Drawing for the job (mm, zero at the part's lowest x, y, z). A direction names the side the tool comes from. Give positions to 0.01 mm unless a question says otherwise; leave off trailing zeros. Order: outer loops, then holes, each group sorted by start corner. A loop starts at its lowest first (then second) coordinate and runs counter-clockwise, first axis right, second up. Notation, with made-up numbers: (22.5, 82) -> (70.5, 82) arc R31 cw to (70.5, 107) -> close; hole circle Ø1 at (69.25, 83). An arc over 180 degrees is marked (long way). Use one line per item in the form item = value. Start each with the question number.
1) Drop flat-ended pins along their axis: P1, Ø3, axis at x = 35.5, z = 35.5, coming from the +Y side; P2, Ø1, axis at y = 1, z = 18.5, coming from the +X side. Give the stop position or say it passes through.
2) Mould opens along X. For the marked faces 1 and 2 say: pulls with the +X half, pulls with the -X half, needs draft (parallel to the pull), parting line crosses it, or undercut.
3) Probe line 1 (Z direction, x = 4.5, y = 1.4) (1 decimal); line 2 (X direction, y = 1.55, z = 3.5); line 3 (X direction, y = 0.65, z = 35.5) (1 decimal). List the from-to ranges inside material, lowest first.
4) Cut at C-C, the plane y = 4.7. Give the cut face in (x, z).
5) Cut at D-D, the plane y = 1.15. Give the cut face in (x, z).
6) Tool access for the marked faces 3, 4 and 5: list every direction of +Z, -Z, +X, -X, +Y, -Y with a clear straight run to the whole face (end or side of a thin tool).
7) Cut at A-A, the plane x = 20. Give the cut face in (y, z), and give its area (3 significant figures).
8) Cut at B-B, the plane z = 20. Give the cut face in (x, y), and give its area (3 significant figures).
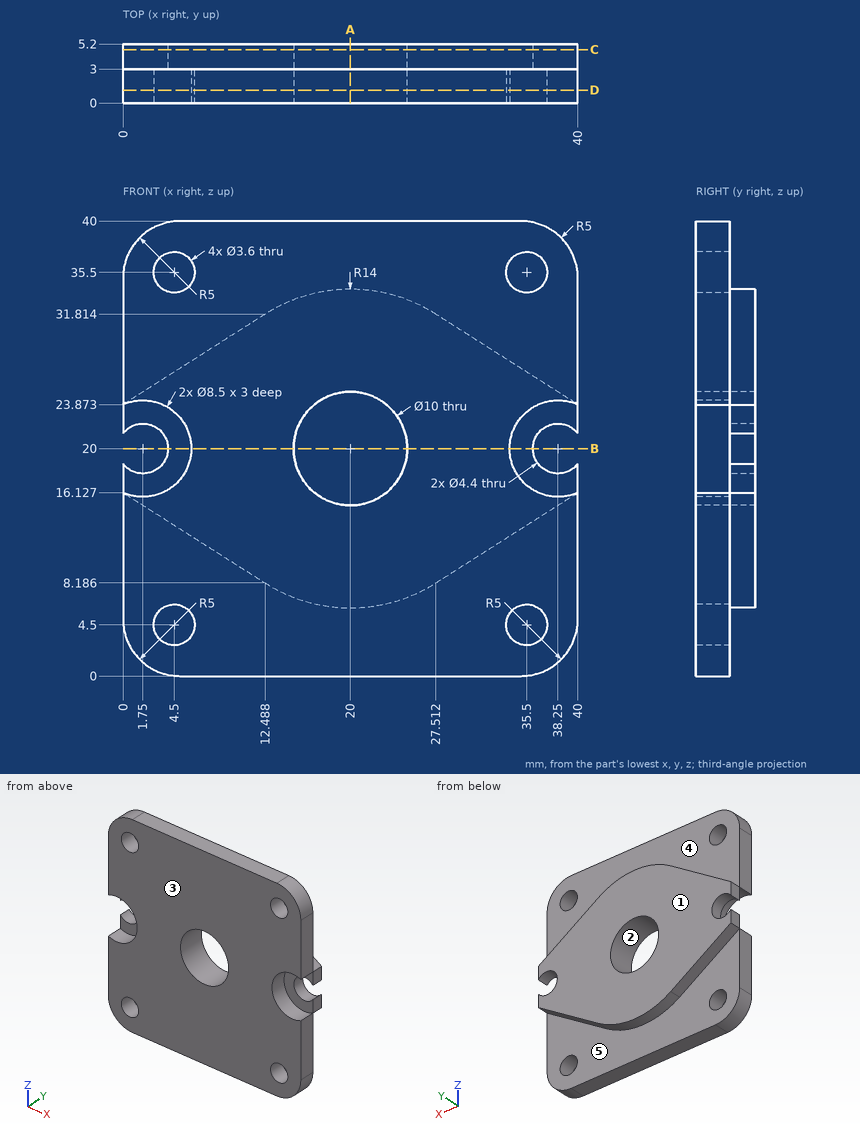
Result:
q1.P1 = through
q1.P2 = 34.5
q2.face_1 = needs draft
q2.face_2 = undercut
q3.line_1 = 0 to 2.7, 6.3 to 16.8, 23.2 to 33.7, 37.3 to 40
q3.line_2 = 0.23 to 3, 6 to 34, 37 to 39.77
q3.line_3 = 0 to 2.7, 6.3 to 33.7, 37.3 to 40
q4.outline = (0, 16.13) -> (12.49, 8.19) arc R14 ccw to (27.51, 8.19) -> (40, 16.13) -> (40, 18.67) arc R2.2 cw (long way) to (40, 21.33) -> (40, 23.87) -> (27.51, 31.81) arc R14 ccw to (12.49, 31.81) -> (0, 23.87) -> (0, 21.33) arc R2.2 cw (long way) to (0, 18.67) -> close; hole circle Ø10 at (20, 20)
q5.outline = (0, 5) arc R5 ccw to (5, 0) -> (35, 0) arc R5 ccw to (40, 5) -> (40, 16.13) arc R4.25 cw (long way) to (40, 23.87) -> (40, 35) arc R5 ccw to (35, 40) -> (5, 40) arc R5 ccw to (0, 35) -> (0, 23.87) arc R4.25 cw (long way) to (0, 16.13) -> close; hole circle Ø3.6 at (4.5, 4.5); hole circle Ø3.6 at (4.5, 35.5); hole circle Ø10 at (20, 20); hole circle Ø3.6 at (35.5, 4.5); hole circle Ø3.6 at (35.5, 35.5)
q6.face_3 = +Z, -Z, +X, -X, -Y
q6.face_4 = +Z, +Y
q6.face_5 = -Z, +Y
q7.outline = (0, 0) -> (3, 0) -> (3, 6) -> (5.2, 6) -> (5.2, 15) -> (0, 15) -> close; (0, 25) -> (5.2, 25) -> (5.2, 34) -> (3, 34) -> (3, 40) -> (0, 40) -> close
q7.area = 130 mm²
q8.outline = (3.95, 3) -> (6, 3) -> (6, 0) -> (15, 0) -> (15, 5.2) -> (3.95, 5.2) -> close; (25, 0) -> (34, 0) -> (34, 3) -> (36.05, 3) -> (36.05, 5.2) -> (25, 5.2) -> close
q8.area = 103 mm²
